Can you work these out from the model? Positions are in its coordinate system, mm. A direction names the side the tool comes from. Coordinates: 2 decimals unless noted, no trailing zeros. Loops run counter-clockwise (first coordinate to the right, second up) from the corner with the lowest first, then second, coordinate; pieces in that order, holes last. Notation, with made-up numbers: (12, 3.25) -> (68, 3.25) arc R16 ccw to (68, 28.25) -> close; hole circle Ø9 at (-34.75, 45.25). An arc over 180 degrees is marked (long way). Use one line per item in the form item = value. Start each with the question number.
(1) Imagine slicing it at A-A (x = 0). List the corners of the cut face in (y, z) for me, plus the area to 3 significant figures.
(2) I need wall thicknesses on line 1 (Y direction, x = 0, z = 0.6); line 2 (Y direction, x = 1.75, z = 0.7); line 3 (X direction, y = -46, z = 0.35). Which ranges of each line are inside material? Lowest first, please. Write a range as [from, to].
(3) Imagine slicing it at D-D (y = -45). List the corners of the cut face in (x, z) for me, plus the area to 3 significant figures.
(4) Imagine slicing it at C-C (y = 1.5). List the corners of the cut face in (x, z) for me, plus the area to 3 significant figures.
(5) On a 3-axis mill with a long thin cutter (end or side, diameter ignored), from which of +Z, -Z, +X, -X, +Y, -Y can I reach the whole of each face in a straight line? I mean faces 1 (the cylindrical face through (2.994, -0.186, 0.444)), 2 (the cylindrical face through (2.01, 5.2, 0.46)). Say none if no direction works.
(6) Thinking about a two-plate mould opening in X: for faces 3 (the flat face through (0, -26, 0.9)), 4 (the cylindrical face through (0.03, -8.54, 0.44)), 5 (the cylindrical face through (-5.576, 2.215, 0.444)), which applies, released by +X, released by -X, zero draft, split by the parting line, or undercut?
(7) Imagine slicing it at B-B (z = 0.7). List the corners of the cut face in (x, y) for me (1 decimal).
```python
from build123d import *

# Parameters (mm, degrees)
ESQUISSE1_R        = 3
BOSS_EXTRU_1_DEPTH = 0.9
CONG_1_R           = 15
CONG_2_R           = 1


with BuildPart() as part:
    # Esquisse1 → Boss.-Extru.1 (new body)
    with BuildSketch(Plane.XY):
        with BuildLine():
            Line((-1.5, 2.598076211), (-1.5, 5.809475019))
            ThreePointArc((-1.5, 5.809475019), (-5.602135703, 2.148505426), (-5, -3.31662479))
            Line((-5, -3.31662479), (-5, -53.31662479))
            ThreePointArc((-5, -53.31662479), (0, -58.31662479), (5, -53.31662479))
            Line((5, -53.31662479), (5, -3.31662479))
            ThreePointArc((5, -3.31662479), (5.602135703, 2.148505426), (1.5, 5.809475019))
            Line((1.5, 5.809475019), (1.5, 2.598076211))
            ThreePointArc((1.5, 2.598076211), (3, 0), (1.5, -2.598076211))
            Line((1.5, -2.598076211), (1.5, -7.04210447))
            ThreePointArc((1.5, -7.04210447), (0, -8.54210447), (-1.5, -7.04210447))
            Line((-1.5, -7.04210447), (-1.5, -2.598076211))
            ThreePointArc((-1.5, -2.598076211), (-3, 0), (-1.5, 2.598076211))
        make_face()
        with Locations((0, -53.31662479)):
            Circle(ESQUISSE1_R, mode=Mode.SUBTRACT)
    extrude(amount=BOSS_EXTRU_1_DEPTH)

    # Congé1
    cong_1_edges = [part.edges().sort_by_distance(p)[0] for p in [
        (5, -3.31662479, 0.45),
        (-5, -3.31662479, 0.45),
    ]]
    fillet(cong_1_edges, radius=CONG_1_R)

    # Congé2
    cong_2_edges = [part.edges().sort_by_distance(p)[0] for p in [
        (1.5, 2.598076211, 0.45),
        (1.5, 5.809475019, 0.45),
        (-1.5, 5.809475019, 0.45),
        (-1.5, 2.598076211, 0.45),
    ]]
    fillet(cong_2_edges, radius=CONG_2_R)


solid = part.part
```
Worked out:
q1.outline = (-58.32, 0) -> (-56.32, 0) -> (-56.32, 0.9) -> (-58.32, 0.9) -> close; (-50.32, 0) -> (-8.54, 0) -> (-8.54, 0.9) -> (-50.32, 0.9) -> close
q1.area = 39.4 mm2
q2.line_1 = [-58.32, -56.32], [-50.32, -8.54]
q2.line_2 = [-58, -55.75], [-50.88, -2.44], [2.46, 4.99]
q2.line_3 = [-5, 5]
q3.outline = (-5, 0) -> (5, 0) -> (5, 0.9) -> (-5, 0.9) -> close
q3.area = 9.00 mm2
q4.outline = (-5.81, 0) -> (-2.6, 0) -> (-2.6, 0.9) -> (-5.81, 0.9) -> close; (2.6, 0) -> (5.81, 0) -> (5.81, 0.9) -> (2.6, 0.9) -> close
q4.area = 5.78 mm2
q5.face_1 = +Z, -Z
q5.face_2 = +Z, -Z, +Y
q6.face_3 = zero draft
q6.face_4 = undercut
q6.face_5 = released by -X
q7.outline = (-5.7, -1.8) arc R15 cw to (-5, -6.4) -> (-5, -53.3) arc R5 ccw to (5, -53.3) -> (5, -6.4) arc R15 cw to (5.7, -1.8) arc R6 ccw to (3, 5.2) arc R1 ccw to (1.5, 4.3) -> (1.5, 3.1) arc R1 ccw to (1.9, 2.3) arc R3 cw to (1.5, -2.6) -> (1.5, -7) arc R1.5 cw to (-1.5, -7) -> (-1.5, -2.6) arc R3 cw to (-1.9, 2.3) arc R1 ccw to (-1.5, 3.1) -> (-1.5, 4.3) arc R1 ccw to (-3, 5.2) arc R6 ccw to start; hole circle Ø6 at (0, -53.3)
